```python
from build123d import *

# Parameters (mm, degrees)
F1_R     = 21.844
F2_DEPTH = 3.175
F3_R     = 28.575
F4_DEPTH = 3.175
F6_DEPTH = 3.175


# Not quite as in the source:
# - a variable given as a bare number and used for a length is read in inches; the dataset says mm whatever the document's units were


with BuildPart() as f2:
    # F1 (on Front) → F2 (new body)
    with BuildSketch(Plane.XZ):
        with BuildLine():
            Line((33.3375, 0), (33.3375, 44.45))
            ThreePointArc((33.3375, 44.45), (0, 77.7875), (-33.3375, 44.45))
            Line((-33.3375, 44.45), (-33.3375, 0))
            Line((-33.3375, 0), (33.3375, 0))
        make_face()
        with Locations((0, 44.45)):
            Circle(F1_R, mode=Mode.SUBTRACT)
    extrude(amount=F2_DEPTH)

    # F3 (on face) → F4 (join)
    with BuildSketch(Plane(origin=(0, 0, 0), x_dir=(1, 0, 0), z_dir=(0, 0, -1))):
        with BuildLine():
            Line((-33.3375, 38.1), (-33.3375, 3.175))
            Line((-33.3375, 3.175), (33.3375, 3.175))
            Line((33.3375, 3.175), (33.3375, 38.1))
            ThreePointArc((33.3375, 38.1), (0, 71.4375), (-33.3375, 38.1))
        make_face()
        with Locations((0, 38.1)):
            Circle(F3_R, mode=Mode.SUBTRACT)
    extrude(amount=-F4_DEPTH)

    # F5 (on face) → F6 (join)
    with BuildSketch(Plane.YZ.offset(33.3375)):
        Polygon((-3.175, 3.175), (-3.175, 28.575), (-28.575, 3.175), align=None)
    extrude(amount=-F6_DEPTH)

    # F7: F2 across plane


with BuildPart() as f2_1:
    add(f2.part)
    add(f2.part.mirror(Plane.YZ))


solid = f2_1.part
```
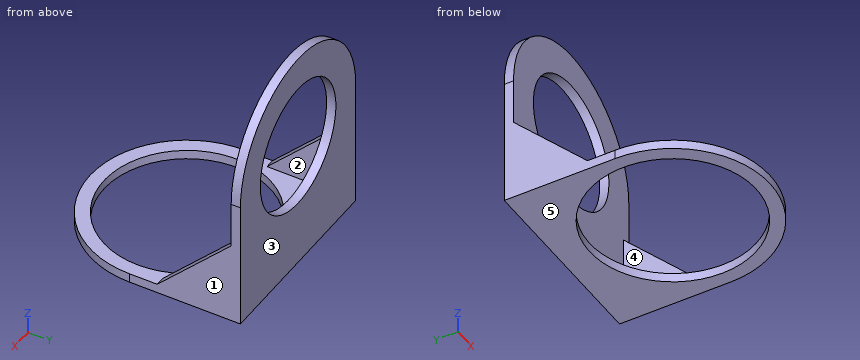
Verification items for the finished model (mm, model axes). Face numbers are marked on the shaded views. A direction names the side the tool comes from. Give positions to 0.01 mm unless a question says otherwise; leave off trailing zeros. Order: outer loops, then holes, each group sorted by start corner. A loop starts at its lowest first (then second) coordinate and runs counter-clockwise, first axis right, second up. Notation, with made-up numbers: (-1.5, 83.5) - (12.5, 83.5) arc R28 ccw to (12.5, 103.5) - close; hole circle Ø7 at (-29.75, -26). An arc over 180 degrees is marked (long way). Answer as CSV lines item,"result". Start each with the question number.
Item 1: Mould release check, pull along X, two halves, no side actions. Record for the marked faces 1, 2 and 3: released by +X, released by -X, zero draft, split by the parting line, or undercut.
Item 2: Access from +Z, -Z, +X, -X, +Y, -Y to the whole of each face (thin tool, end or side, straight path). Record for the marked faces 4 and 5.
Item 3: Material ranges on L1, parallel to Z at x = 0, y = -1.6; L2, parallel to Y at x = 0, z = 2.05 (1 decimal); L3, parallel to Y at x = -14.5, z = 67.5 (3 decimals), recorded low to high.
Item 4: Section check D-D, the plane z = 40. Record the boundary of the cut face in (x, y) (1 decimal), plus the area to 3 significant figures.
Item 5: Gauge pin test, flat ends, axial feed: pin 1 (5 mm diameter, centred on x = 25.5, y = -15.5, fed in from +Z) (3 decimals); pin 2 (4 mm diameter, centred on x = -3.5, z = 67.5, fed in from -Y) (3 decimals); pin 3 (20.5 mm diameter, centred on y = -22, z = 22, fed in from +X). Record the tip position at first contact, or that the pin passes through.
Item 6: Section check A-A, the plane x = 0. Record the boundary of the cut face in (y, z) (1 decimal), plus the area to 3 significant figures.
Filled in:
1,face 1,"released by +X"
1,face 2,"undercut"
1,face 3,"zero draft"
2,face 4,"+Z, -Y"
2,face 5,"-Z, +X, -X, +Y, -Y"
3,L1,"0 to 22.61, 66.29 to 77.79"
3,L2,"-71.4 to -66.7, -9.5 to 0"
3,L3,"-3.175 to 0"
4,outline,"(-33.3, -3.2) - (-21.4, -3.2) - (-21.4, 0) - (-33.3, 0) - close; (21.4, -3.2) - (33.3, -3.2) - (33.3, 0) - (21.4, 0) - close"
4,area,"75.9 mm^2"
5,pin 1,"z = 3.175"
5,pin 2,"y = -3.175"
5,pin 3,"x = 33.34"
6,outline,"(-71.4, 0) - (-66.7, 0) - (-66.7, 3.2) - (-71.4, 3.2) - close; (-9.5, 0) - (0, 0) - (0, 22.6) - (-3.2, 22.6) - (-3.2, 3.2) - (-9.5, 3.2) - close; (-3.2, 66.3) - (0, 66.3) - (0, 77.8) - (-3.2, 77.8) - close"
6,area,"144 mm^2"
